CAD build for the part. Positions are in the model's coordinates, mm. Coordinates: 2 decimals unless noted, no trailing zeros. Order: outer loops, then holes, each group sorted by start corner. A loop starts at its lowest first (then second) coordinate and runs counter-clockwise, first axis right, second up.
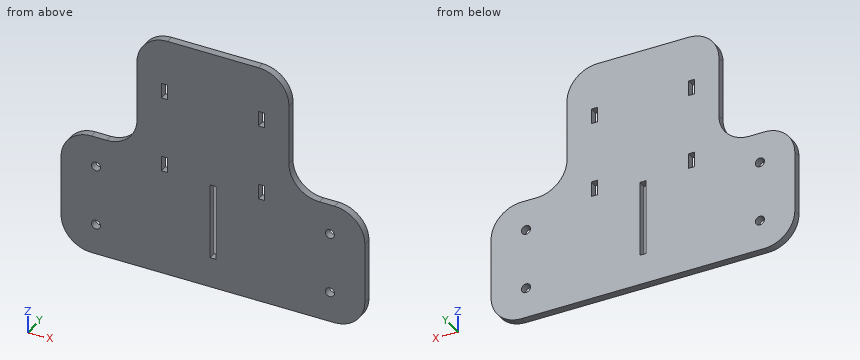
from build123d import *

# Parameters (mm, degrees)
SKETCH1_R           = 1.5
SKETCH1_W           = 2
SKETCH1_H           = 5
SKETCH1_H_2         = 25
BOSS_EXTRUDE1_DEPTH = 1.25
FILLET1_R           = 10


with BuildPart() as part:
    # Sketch1 → Boss-Extrude1 (new, symmetric)
    with BuildSketch(Plane(origin=(0, 0, 0), x_dir=(1, 0, 0), z_dir=(0, 1, 0))):
        Polygon((-50, 40), (50, 40), (50, 0), (25, 0), (25, -40), (-25, -40), (-25, 0), (-50, 0), align=None)
        with Locations(Location((-38.5, 30, 0), (0, 0, 270))):
            Circle(SKETCH1_R, mode=Mode.SUBTRACT)
        with Locations(Location((38.5, 30, 0), (0, 0, 90))):
            Circle(SKETCH1_R, mode=Mode.SUBTRACT)
        with Locations(Location((-38.5, 10, 0), (0, 0, 270))):
            Circle(SKETCH1_R, mode=Mode.SUBTRACT)
        with Locations(Location((38.5, 10, 0), (0, 0, 90))):
            Circle(SKETCH1_R, mode=Mode.SUBTRACT)
        with Locations((16, -22.5)):
            Rectangle(SKETCH1_W, SKETCH1_H, mode=Mode.SUBTRACT)
        with Locations((-16, -22.5)):
            Rectangle(SKETCH1_W, SKETCH1_H, mode=Mode.SUBTRACT)
        with Locations((-16, 2.5)):
            Rectangle(SKETCH1_W, SKETCH1_H, mode=Mode.SUBTRACT)
        with Locations((16, 2.5)):
            Rectangle(SKETCH1_W, SKETCH1_H, mode=Mode.SUBTRACT)
        with Locations((0, 17.5)):
            Rectangle(SKETCH1_W, SKETCH1_H_2, mode=Mode.SUBTRACT)
    extrude(amount=BOSS_EXTRUDE1_DEPTH, both=True)

    # Fillet1
    fillet1_edges = [part.edges().sort_by_distance(p)[0] for p in [
        (50, 0, 0),
        (25, 0, 0),
        (25, 0, 40),
        (-25, 0, 40),
        (-25, 0, 0),
        (-50, 0, 0),
        (-50, 0, -40),
        (50, 0, -40),
    ]]
    fillet(fillet1_edges, radius=FILLET1_R)


solid = part.part
1) Slice it at D-D (z = -6.5). List the corners of the cut face in (x, y).
2) Slice it at C-C (y = -0.5). Give the number of separate pieces and of enclosed holes in the cut face, plus the area to 3 significant figures.
3) Pin check, flat tips, straight feed: P1, Ø0.8, axis at y = 0, z = -2, coming from the +X side; P2, Ø1.5, axis at x = -24, y = -1, coming from the +Z side; P3, Ø0.6, axis at x = 15.5, y = 0.5, coming from the +Z side. Stop position of each tip, or through.
4) Slice it at B-B (x = -38.5). List the corners of the cut face in (y, z), plus the area to 3 significant figures.
5) Drill centre lines: probe 1 along X at (y, z) = (0.5, 23); probe 2 along Z at (x, y) = (38.5, -0.55); probe 3 along X at (y, z) = (-0.95, -25). Where is each one in solid material? Low to high.
6) Slice it at A-A (z = -27). List the corners of the cut face in (x, y).
Worked out:
1. outline: (-49.37, -1.25) - (-1, -1.25) - (-1, 1.25) - (-49.37, 1.25) - close; (1, -1.25) - (49.37, -1.25) - (49.37, 1.25) - (1, 1.25) - close
2. separate pieces: 1
2. enclosed holes: 9
2. area: 5,800 mm2
3. P1: stops at x = 46.5
3. P2: stops at z = 35.65
3. P3: stops at z = 40
4. outline: (-1.25, -40) - (1.25, -40) - (1.25, -31.5) - (-1.25, -31.5) - close; (-1.25, -28.5) - (1.25, -28.5) - (1.25, -11.5) - (-1.25, -11.5) - close; (-1.25, -8.5) - (1.25, -8.5) - (1.25, 0) - (-1.25, 0) - close
4. area: 85.0 mm2
5. probe 1: x = -25 to -17, -15 to 15, 17 to 25
5. probe 2: z = -40 to -31.5, -28.5 to -11.5, -8.5 to 0
5. probe 3: x = -50 to -1, 1 to 50
6. outline: (-50, -1.25) - (-1, -1.25) - (-1, 1.25) - (-50, 1.25) - close; (1, -1.25) - (50, -1.25) - (50, 1.25) - (1, 1.25) - close
